Read the model definition and answer for the solid it produces. Units are mm, in the model's axes. A direction names the side the tool comes from. Coordinates: 2 decimals unless noted, no trailing zeros. Order: outer loops, then holes, each group sorted by start corner. A loop starts at its lowest first (then second) coordinate and runs counter-clockwise, first axis right, second up. Notation, with made-up numbers: (11, -4) -> (23, -4) arc R10 ccw to (23, 11) -> close; hole circle Ø4 at (85, 46). An arc over 180 degrees is marked (long way). Answer as a JSON object with one key per item and string values. Group by question number.
1) Determine the mould class of faces 3 (the flat face through (1, -1, 0)), 4 (the flat face through (-1, -1, 5.08)), 5 (the flat face through (48, 31.75, 50)), 6 (the cylindrical face through (-43.61, -13.73, 54.02)) for opening direction Y: released by +Y, released by -Y, zero draft, split by the parting line, or undercut.
2) Section B-B on y = -24 is taken. Determine the outline of the cut face in (x, z), and give its area (3 significant figures).
3) Given pin 1 (3 mm diameter, centred on y = 10, z = 39, fed in from -X); pin 2 (12 mm diameter, centred on y = 11, z = 43, fed in from -X); pin 3 (3 mm diameter, centred on x = -32.5, y = -20.5, fed in from -Z); pin 4 (2.5 mm diameter, centred on x = 48, z = 31.5, fed in from -Y), each flat-ended and moving along its own axis, determine where each tip first touches the part or whether it passes through.
4) Section A-A on z = 44 is taken. Determine the outline of the cut face in (x, y).
5) Section C-C on y = 0 is taken. Determine the outline of the cut face in (x, z), and give its area (3 significant figures).
6) Consider L1, parallel to Y at x = 0, z = 49; L2, parallel to X at y = 24, z = 78.5; L3, parallel to Z at x = -40, y = 16. Determine where each line is inside the solid, lowest interval first.
7) A tool of negligible diameter and unlimited length cuts with its end or side. For faces 1 (the flat face through (48, -31.75, 50)), 2 (the flat face through (45.4, -7.8, 101.6)), from which of +Z, -Z, +X, -X, +Y, -Y can it reach the whole face along a straight path? Write none if from no direction.
from build123d import *

# Parameters (mm, degrees)
F4_W     = 63.5
F4_H     = 101.6
F5_DEPTH = 5.08


with BuildPart() as f2:
    # F0 (on Front) → F2 (revolve)
    with BuildSketch(Plane.XZ):
        Polygon((-45.72, 101.6), (-50.8, 101.6), (-50.8, 0), (-45.72, 0), (0, 0), (0, 5.08), (-45.72, 5.08), align=None)
    revolve(axis=Axis((0, 0, 36.652558), (0, 0, 1)))

    # F4 (on offset) → F5 (join)
    with BuildSketch(Plane.YZ.offset(50.8)):
        with Locations((0, 50.8)):
            Rectangle(F4_W, F4_H)
    extrude(amount=-F5_DEPTH)


solid = f2.part
Worked answers:
{
 "1": {"face 3": "zero draft", "face 4": "undercut", "face 5": "released by +Y", "face 6": "undercut"},
 "2": {"outline": "(-44.77, 0) -> (44.77, 0) -> (44.77, 101.6) -> (38.91, 101.6) -> (38.91, 5.08) -> (-38.91, 5.08) -> (-38.91, 101.6) -> (-44.77, 101.6) -> close; (45.72, 0) -> (50.8, 0) -> (50.8, 101.6) -> (45.72, 101.6) -> close", "area": "2,100 mm²"},
 "3": {"pin 1": "stops at x = -50.08", "pin 2": "stops at x = -50.55", "pin 3": "stops at z = 0", "pin 4": "stops at y = -31.75"},
 "4": {"outline": "(45.72, -31.75) -> (50.8, -31.75) -> (50.8, 31.75) -> (45.72, 31.75) -> (45.72, 22.14) arc R50.8 ccw (long way) to (45.72, -22.14) -> close; hole circle Ø91.44 at (0, 0)"},
 "5": {"outline": "(-50.8, 0) -> (50.8, 0) -> (50.8, 101.6) -> (45.72, 101.6) -> (45.72, 5.08) -> (-45.72, 5.08) -> (-45.72, 101.6) -> (-50.8, 101.6) -> close", "area": "1,500 mm²"},
 "6": {"L1": "y = -50.8 to -45.72, 45.72 to 50.8", "L2": "x = -44.77 to -38.91, 38.91 to 44.77, 45.72 to 50.8", "L3": "z = 0 to 5.08"},
 "7": {"face 1": "+Z, -Z, +X, -Y", "face 2": "+Z, +X, -X, +Y, -Y"}
}
